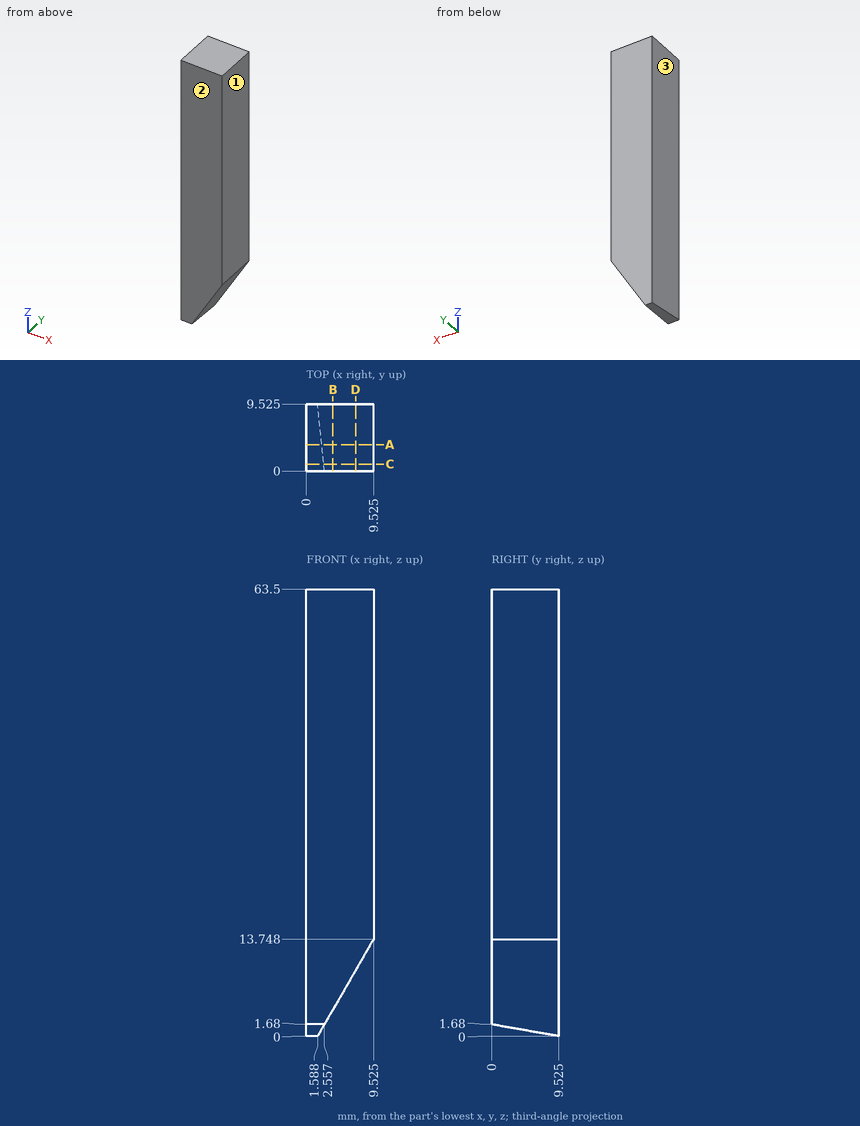
Answer from the drawing. Dimensions are ordinates in mm from the lowest x, y and z of the part. Round coordinates to 2 decimals unless told otherwise and drop trailing zeros. Write each loop counter-clockwise with the first axis right and the second up, starting at its lowest first coordinate (ties: lowest second). Pieces come first, ordered by that corner, then holes. Notation, with made-up numbers: M -36.5,-9.5 L 0.5,-9.5 A19 ccw 0.5,14.5 Z; hole C 21.25,37.5 d5. An arc over 180 degrees is marked long. Write each question's results on one line, items separated by ' | '. Start each with the question number.
Item 1: Given pin 1 Ø1 at (y, z) = (4, 13) entering from +X, flat-ended and moving along its own axis, determine where the tip first touches the part or whether it passes through.
Item 2: Find section C-C on y = 1. Write down the section's boundary in (x, z) (1 decimal), and give its area (3 significant figures).
Item 3: Find section D-D on x = 7. Write down the section's boundary in (y, z) (1 decimal).
Item 4: Straight lines are drawn through the part: probe 1 along X at (y, z) = (0.5, 4.5) (1 decimal); probe 2 along Z at (x, y) = (8.75, 3.25) (1 decimal); probe 3 along Z at (x, y) = (8.25, 4.5). For each, find the intervals that lie inside material, in ascending order.
Item 5: Find section A-A on y = 3.75. Write down the section's boundary in (x, z) (1 decimal).
Item 6: The mould has two halves that part along X. Classify the marked faces 1, 2 and 3: +X half, -X half, draft (parallel to the pull), parting line (faces both ways), or undercut.
Item 7: Find section B-B on x = 3.75. Write down the section's boundary in (y, z) (1 decimal), and give its area (3 significant figures).
Answer block:
1) pin 1: stops at x = 9.38
2) outline: M 0,1.5 L 2.5,1.5 L 9.5,13.7 L 9.5,63.5 L 0,63.5 Z | area: 547 mm²
3) outline: M 0,9.4 L 9.5,9.4 L 9.5,63.5 L 0,63.5 Z
4) probe 1: x = 0 to 4.2 | probe 2: z = 12.4 to 63.5 | probe 3: z = 11.54 to 63.5
5) outline: M 0,1 L 2.2,1 L 9.5,13.7 L 9.5,63.5 L 0,63.5 Z
6) face 1: +X half | face 2: draft | face 3: -X half
7) outline: M 0,3.7 L 9.5,3.7 L 9.5,63.5 L 0,63.5 Z | area: 569 mm²
